```python
from build123d import *

# Parameters (mm, degrees)
SKETCH1_R           = 10.89504564
BOSS_EXTRUDE1_DEPTH = 38.1
BOSS_EXTRUDE2_DEPTH = 8.89
SKETCH3_W           = 63.5
SKETCH3_H           = 6.927272727
BOSS_EXTRUDE3_DEPTH = 38.1
BOSS_EXTRUDE4_DEPTH = 38.1
FILLET1_R           = 6.35


with BuildPart() as part:
    # Sketch1 → Boss-Extrude1 (new body)
    with BuildSketch(Plane.XY):
        Circle(SKETCH1_R)
    extrude(amount=-BOSS_EXTRUDE1_DEPTH)

    # Sketch2 → Boss-Extrude2 (add)
    with BuildSketch(Plane(origin=(0, 0, -38.1), x_dir=(-1, 0, 0), z_dir=(0, 0, -1))):
        Polygon((-11.176, 0), (11.176, 0), (22.604396494, 19.05), (11.176, 19.05), (-11.176, 19.05), (-22.604396494, 19.05), align=None)
    extrude(amount=-BOSS_EXTRUDE2_DEPTH)

    # Sketch3 → Boss-Extrude3 (add)
    with BuildSketch(Plane(origin=(0, 0, -38.1), x_dir=(-1, 0, 0), z_dir=(0, 0, -1))):
        with Locations((0, 22.513636364)):
            Rectangle(SKETCH3_W, SKETCH3_H)
    extrude(amount=-BOSS_EXTRUDE3_DEPTH)

    # Sketch4 → Boss-Extrude4 (add)
    with BuildSketch(Plane(origin=(0, 0, -38.1), x_dir=(-1, 0, 0), z_dir=(0, 0, -1))):
        Polygon((-31.75, 25.977272727), (-31.75, 64.077272727), (-6.35, 64.077272727), (-6.35, 76.777272727), (-35.948347107, 76.777272727), (-35.948347107, 19.05), (-31.75, 19.05), align=None)
        Polygon((31.75, 25.977272727), (31.75, 64.077272727), (6.35, 64.077272727), (6.35, 76.777272727), (35.948347107, 76.777272727), (35.948347107, 19.05), (31.75, 19.05), align=None)
    extrude(amount=-BOSS_EXTRUDE4_DEPTH)

    # Fillet1
    fillet1_edges = [part.edges().sort_by_distance(p)[0] for p in [
        (35.948347107, 19.05, -19.05),
        (35.948347107, 76.777272727, -19.05),
        (-35.948347107, 76.777272727, -19.05),
        (-35.948347107, 19.05, -19.05),
    ]]
    fillet(fillet1_edges, radius=FILLET1_R)


solid = part.part
```
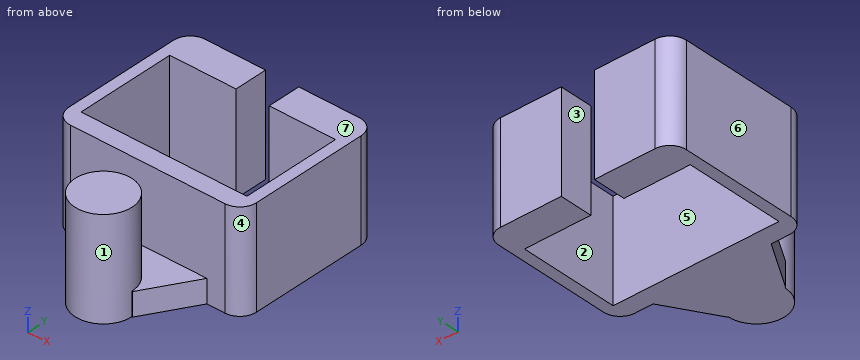
Part model, mm, in its own coordinate system. Face numbers are marked on the shaded views. A direction names the side the tool comes from. Round coordinates to 2 decimals unless told otherwise and drop trailing zeros. Order: outer loops, then holes, each group sorted by start corner. A loop starts at its lowest first (then second) coordinate and runs counter-clockwise, first axis right, second up. Notation, with made-up numbers: M 36,43 L 43,43 A7 cw 43,53 Z; hole C 39,77 d1. An arc over 180 degrees is marked long. Answer in a Markdown table with one row per item. Add a question column.
Q1. Wall check: L1, parallel to X at y = 47.5, z = -3; L2, parallel to Y at x = -24, z = -12; L3, parallel to X at y = 69, z = -36. Give the ranges that are in metal, low to high. Write a range as from..to.
Q2. Mould opens along X. For the marked faces 5, 6 and 7 say: +X half, -X half, draft (parallel to the pull), parting line (faces both ways), or undercut.
Q3. Pin check, flat tips, straight feed: pin 1 (2 mm diameter, centred on x = 13, y = 21, fed in from +Z); pin 2 (20.5 mm diameter, centred on x = -15.5, z = -27.5, fed in from -Y); pin 3 (5.5 mm diameter, centred on x = 4, y = 14.5, fed in from +Z); pin 4 (7.5 mm diameter, centred on x = 22, z = -13, fed in from -Y). Stop position of each tip, or through.
Q4. Cut at C-C on x = -15.5. Give the cut face in (y, z), and give its area (3 significant figures).
Q5. Cut at A-A on y = 69. Give the cut face in (x, z).
Q6. 3-axis set-ups, long thin cutter, end or side, ignore diameter. For the marked faces 1, 2, 3 and 4: which of +Z, -Z, +X, -X, +Y, -Y reach the whole face in a straight line?
Q7. Cut at D-D on x = 0. Give the cut face in (y, z).
Q8. Cut at B-B on z = -7. Give the cut face in (x, y), and give its area (3 significant figures).
Established:
| question | item | result |
|---|---|---|
| 1 | L1 | x = -35.95..-31.75, 31.75..35.95 |
| 1 | L2 | y = 19.05..25.98, 64.08..76.78 |
| 1 | L3 | x = -35.95..-6.35, 6.35..35.95 |
| 2 | face 5 | undercut |
| 2 | face 6 | -X half |
| 2 | face 7 | draft |
| 3 | pin 1 | stops at z = 0 |
| 3 | pin 2 | stops at y = -9.55 |
| 3 | pin 3 | stops at z = -29.21 |
| 3 | pin 4 | stops at y = 19.05 |
| 4 | outline | M 7.21,-38.1 L 25.98,-38.1 L 25.98,0 L 19.05,0 L 19.05,-29.21 L 7.21,-29.21 Z; M 64.08,-38.1 L 76.78,-38.1 L 76.78,0 L 64.08,0 Z |
| 4 | area | 853 mm2 |
| 5 | outline | M -35.95,-38.1 L -6.35,-38.1 L -6.35,0 L -35.95,0 Z; M 6.35,-38.1 L 35.95,-38.1 L 35.95,0 L 6.35,0 Z |
| 6 | face 1 | +Z |
| 6 | face 2 | +Z, -Z |
| 6 | face 3 | +Z, -Z, +Y |
| 6 | face 4 | +Z, -Z, +X, -Y |
| 7 | outline | M -10.9,-38.1 L 25.98,-38.1 L 25.98,0 L 19.05,0 L 19.05,-29.21 L 10.9,-29.21 L 10.9,0 L -10.9,0 Z |
| 8 | outline | M -35.95,25.4 A6.35 ccw -29.6,19.05 L 29.6,19.05 A6.35 ccw 35.95,25.4 L 35.95,70.43 A6.35 ccw 29.6,76.78 L 6.35,76.78 L 6.35,64.08 L 31.75,64.08 L 31.75,25.98 L -31.75,25.98 L -31.75,64.08 L -6.35,64.08 L -6.35,76.78 L -29.6,76.78 A6.35 ccw -35.95,70.43 Z; C 0,0 d21.79 |
| 8 | area | 1,910 mm2 |
